```python
from build123d import *

# Parameters (mm, degrees)
F0_W      = 13
F0_H      = 28
F1_DEPTH  = 1.5
F2_W      = 1.75
F2_H      = 3
F2_W_2    = 0.25
F3_DEPTH  = 25
F4_W      = 2.6
F4_H      = 2.6
F5_DEPTH  = 0.05
F6_R      = 0.2
F7_R      = 0.24999
F8_W      = 2.6
F8_H      = 2.6
F9_DEPTH  = 0.05
F10_R     = 0.2
F11_W     = 3.6
F11_H     = 3.6
F12_DEPTH = 1.25
F13_W     = 7
F13_H     = 7
F14_DEPTH = 1.25


# Not quite as in the source:
# - a fillet or chamfer is up to 0.001 mm smaller than in the source, because OpenCascade refuses the exact size


with BuildPart() as f1:
    # F0 (on Top) → F1 (new body)
    with BuildSketch(Plane.XY):
        Rectangle(F0_W, F0_H)
    extrude(amount=F1_DEPTH)

    # F2 (on face) → F3 (cut)
    with BuildSketch(Plane.XY.offset(1.5)):
        with Locations((-2.375, 12.5)):
            Rectangle(F2_W, F2_H)
        with Locations((2.375, 12.5)):
            Rectangle(F2_W, F2_H)
        with Locations((-6.375, 12.5)):
            Rectangle(F2_W_2, F2_H)
        with Locations((6.375, 12.5)):
            Rectangle(F2_W_2, F2_H)
    extrude(amount=-F3_DEPTH, mode=Mode.SUBTRACT)

    # F4 (on face) → F5 (join)
    with BuildSketch(Plane.XY.offset(1.5)):
        with Locations((-4.75, 12.5)):
            Rectangle(F4_W, F4_H)
        with Locations((0, 12.5)):
            Rectangle(F4_W, F4_H)
        with Locations((4.75, 12.5)):
            Rectangle(F4_W, F4_H)
    extrude(amount=F5_DEPTH)

    # F6
    f6_edges = [f1.edges().sort_by_distance(p)[0] for p in [
        (-6.05, 11.2, 1.525),
        (-6.05, 13.8, 1.525),
        (-3.45, 11.2, 1.525),
        (-3.45, 13.8, 1.525),
        (1.3, 13.8, 1.525),
        (-1.3, 13.8, 1.525),
        (1.3, 11.2, 1.525),
        (3.45, 13.8, 1.525),
        (6.05, 13.8, 1.525),
        (6.05, 11.2, 1.525),
        (-1.3, 11.2, 1.525),
        (3.45, 11.2, 1.525),
    ]]
    fillet(f6_edges, radius=F6_R)

    # F7 (radius 0.25 in the source; OpenCascade refuses exactly that, so slightly less here)
    f7_edges = [f1.edges().sort_by_distance(p)[0] for p in [
        (6.25, 11, 0.75),
        (-6.25, 11, 0.75),
        (-1.5, 11, 0.75),
        (3.25, 11, 0.75),
        (-3.25, 11, 0.75),
        (1.5, 11, 0.75),
    ]]
    fillet(f7_edges, radius=F7_R)

    # F8 (on face) → F9 (join)
    with BuildSketch(Plane.XY.offset(1.5)):
        with Locations((-4.8, -12.3)):
            Rectangle(F8_W, F8_H)
        with Locations((4.8, -12.3)):
            Rectangle(F8_W, F8_H)
    extrude(amount=F9_DEPTH)

    # F10
    f10_edges = [f1.edges().sort_by_distance(p)[0] for p in [
        (-6.1, -13.6, 1.525),
        (-3.5, -13.6, 1.525),
        (-6.1, -11, 1.525),
        (3.5, -13.6, 1.525),
        (6.1, -13.6, 1.525),
        (3.5, -11, 1.525),
        (-3.5, -11, 1.525),
        (6.1, -11, 1.525),
    ]]
    fillet(f10_edges, radius=F10_R)

    # F11 (on face) → F12 (join)
    with BuildSketch(Plane.XY.offset(1.5)):
        with Locations((-4.45, 8.95)):
            Rectangle(F11_W, F11_H)
        with Locations((0, 8.95)):
            Rectangle(F11_W, F11_H)
        with Locations((4.45, 8.95)):
            Rectangle(F11_W, F11_H)
        with Locations((4.45, 4.7)):
            Rectangle(F11_W, F11_H)
        with Locations((0, 4.7)):
            Rectangle(F11_W, F11_H)
        with Locations((-4.45, 4.7)):
            Rectangle(F11_W, F11_H)
        with Locations((4.45, 0.45)):
            Rectangle(F11_W, F11_H)
        with Locations((0, 0.45)):
            Rectangle(F11_W, F11_H)
        with Locations((-4.45, 0.45)):
            Rectangle(F11_W, F11_H)
    extrude(amount=F12_DEPTH)

    # F13 (on face) → F14 (join)
    with BuildSketch(Plane(origin=(0, 0, 0), x_dir=(1, 0, 0), z_dir=(0, 0, -1))):
        with Locations((0, -6)):
            Rectangle(F13_W, F13_H)
        with Locations((0, 6)):
            Rectangle(F13_W, F13_H)
    extrude(amount=F14_DEPTH)


solid = f1.part
```
Geometry check sheet. Reference: the model listing, model coordinates, mm. A direction names the side the tool comes from. Coordinates: 2 decimals unless noted, no trailing zeros. Order: outer loops, then holes, each group sorted by start corner. A loop starts at its lowest first (then second) coordinate and runs counter-clockwise, first axis right, second up. Notation, with made-up numbers: (22.25, -10) - (65.25, -10) arc R31 ccw to (65.25, 19) - close; hole circle Ø2 at (86.25, 79). An arc over 180 degrees is marked (long way). Answer in a Markdown table with one row per item. Add a question column.
1. Section check C-C (y = 2). Enter the section's corners in (x, z), plus the area to 3 significant figures.
2. Material ranges on L1, parallel to Y at x = 4.25, z = 2.4; L2, parallel to X at y = 5, z = 2.3; L3, parallel to Y at x = -1, z = -1, recorded low to high. Write a range as [from, to].
3. Section check B-B (x = 4.25). Enter the section's corners in (y, z), plus the area to 3 significant figures.
4. Gauge pin test, flat ends, axial feed: pin 1 Ø0.6 at (y, z) = (-0.5, 2) entering from +X; pin 2 Ø0.6 at (x, z) = (0, 2.5) entering from -Y; pin 3 Ø1.3 at (x, y) = (-5.5, 12) entering from +Z. Record the tip position at first contact, or that the pin passes through.
5. Access from +Z, -Z, +X, -X, +Y, -Y to the whole of each face (thin tool, end or side, straight path). Record for faces 1 (the face through (1.8, 9, 2)), 2 (the face through (-6.25, 13, 1)), 3 (the face through (0, 13, 1.55)), 4 (the face through (0, 6.5, 2)).
6. Section check A-A (z = -0.9). Enter the section's corners in (x, y).
7. Section check D-D (z = 1.9). Give the number of separate pieces and of enclosed holes in the cut face, plus the area to 3 significant figures.
8. Draft check along Y on faces 5 (the face through (4, 0, 2.75)), 6 (the face through (-2, 11, 1)), 7 (the face through (0, 2.9, 2)). Enter one of: +Y half, -Y half, draft (parallel to the pull), parting line (faces both ways), or undercut.
Data:
| question | item | result |
|---|---|---|
| 1 | outline | (-6.5, 0) - (6.5, 0) - (6.5, 1.5) - (6.25, 1.5) - (6.25, 2.75) - (2.65, 2.75) - (2.65, 1.5) - (1.8, 1.5) - (1.8, 2.75) - (-1.8, 2.75) - (-1.8, 1.5) - (-2.65, 1.5) - (-2.65, 2.75) - (-6.25, 2.75) - (-6.25, 1.5) - (-6.5, 1.5) - close |
| 1 | area | 33.0 mm² |
| 2 | L1 | y = [-1.35, 2.25], [2.9, 6.5], [7.15, 10.75] |
| 2 | L2 | x = [-6.25, -2.65], [-1.8, 1.8], [2.65, 6.25] |
| 2 | L3 | y = [-9.5, -2.5], [2.5, 9.5] |
| 3 | outline | (-14, 0) - (14, 0) - (14, 1.5) - (13.8, 1.5) - (13.8, 1.55) - (11.2, 1.55) - (11.2, 1.5) - (10.75, 1.5) - (10.75, 2.75) - (7.15, 2.75) - (7.15, 1.5) - (6.5, 1.5) - (6.5, 2.75) - (2.9, 2.75) - (2.9, 1.5) - (2.25, 1.5) - (2.25, 2.75) - (-1.35, 2.75) - (-1.35, 1.5) - (-11, 1.5) - (-11, 1.55) - (-13.6, 1.55) - (-13.6, 1.5) - (-14, 1.5) - close |
| 3 | area | 55.8 mm² |
| 4 | pin 1 | stops at x = 6.25 |
| 4 | pin 2 | stops at y = -1.35 |
| 4 | pin 3 | stops at z = 1.55 |
| 5 | face 1 | +Z, +Y, -Y |
| 5 | face 2 | +Z, -Z, -X, +Y |
| 5 | face 3 | +Z, +X, -X, +Y |
| 5 | face 4 | +Z, +X, -X |
| 6 | outline | (-3.5, -9.5) - (3.5, -9.5) - (3.5, -2.5) - (-3.5, -2.5) - close; (-3.5, 2.5) - (3.5, 2.5) - (3.5, 9.5) - (-3.5, 9.5) - close |
| 7 | separate pieces | 9 |
| 7 | enclosed holes | 0 |
| 7 | area | 117 mm² |
| 8 | face 5 | draft |
| 8 | face 6 | +Y half |
| 8 | face 7 | undercut |
